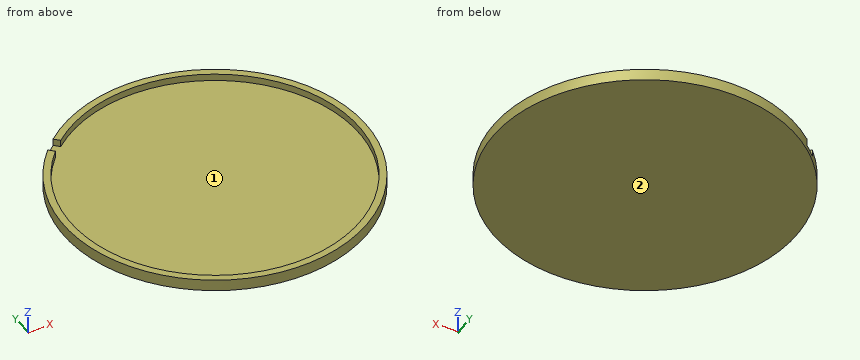
Autodesk Fusion 360 part; units mm, degrees
sketch "Sketch1" plane through (0, 0, 0) normal (0, 0, 1) x (1, 0, 0)
  circle A0 centre (0, 0) radius 65
  dimension "d1" = 130
extrude "Extrude1" add sketch "Sketch1" along normal blind 5
hole "Hole1" at (0, 0, 5) direction (0, 0, -1) diameter 124 depth 3 tip angle 180
sketch "Sketch2" plane through (0, 0, 5) normal (0, 0, 1) x (-1, 0, 0)
  circle A0 centre (0, 0) radius 62
  circle A1 centre (0, 0) radius 65
  line L0 (54.116, -50.8938) -> (49.1662, -55.8435)
  line L1 (49.1662, -55.8435) -> (34.7966, -41.4739)
  line L2 (34.7966, -41.4739) -> (39.7463, -36.5241)
  line L3 (39.7463, -36.5241) -> (54.116, -50.8938)
  dimension "d7" = 7
extrude "Extrude2" cut sketch "Sketch2" against normal blind 3 contours A0 A1 L1 L3 picked at (41.6647, -47.2432)
Can you work these out from the model? Positions are in its coordinate system, mm. Face numbers are marked on the shaded views. Round coordinates to 2 decimals unless told otherwise and drop trailing zeros. Write each loop counter-clockwise with the first axis right and the second up, starting at its lowest first coordinate (ties: lowest second). Pieces come first, ordered by that corner, then holes. Notation, with made-up numbers: M -35.5,15 L 2.5,15 A23 ccw 2.5,26 Z; hole C 36,-30.5 d2. An arc over 180 degrees is marked long. Use a Markdown table: item, result.
Item 1: We'd pull the mould along Y, two halves only. Please class the marked faces 1 and 2: released by +Y, released by -Y, zero draft, split by the parting line, or undercut.
Found:
| item | result |
|---|---|
| face 1 | undercut |
| face 2 | zero draft |
Item 2: I want a section at B-B (x = 35). List the corners of the cut face in (y, z) for me, and give its area (3 significant figures).
Found:
| item | result |
|---|---|
| outline | M -54.77,0 L 54.77,0 L 54.77,5 L 51.18,5 L 51.18,2 L -51.18,2 L -51.18,5 L -54.77,5 Z |
| area | 241 mm2 |
Item 3: For pin 1 Ø2 at (y, z) = (21, 3) entering from +X; pin 2 Ø1 at (x, y) = (28.5, -9) entering from +Z; pin 3 Ø3 at (x, z) = (-43, 1.5) entering from +Y, each with a flat end and sliding along its axis, tell me the tip position at first contact or that it passes through.
Found:
| item | result |
|---|---|
| pin 1 | stops at x = 61.85 |
| pin 2 | stops at z = 2 |
| pin 3 | stops at y = 50.03 |
Item 4: I want a section at A-A (y = 0). List the corners of the cut face in (x, z) for me, and give its area (3 significant figures).
Found:
| item | result |
|---|---|
| outline | M -65,0 L 65,0 L 65,5 L 62,5 L 62,2 L -62,2 L -62,5 L -65,5 Z |
| area | 278 mm2 |
Item 5: If I drill on line 1 along Y through (x, z) = (0.5, 3.95); line 2 along Z through (x, y) = (-29, 47.5), over which ranges is the centre line in solid material (lowest first)? Write a range as [from, to].
Found:
| item | result |
|---|---|
| line 1 | y = [-65, -62], [62, 65] |
| line 2 | z = [0, 2] |
Item 6: I want a section at C-C (z = 2.8). List the corners of the cut face in (x, y) for me.
Found:
| item | result |
|---|---|
| outline | M -47.54,44.32 A65 ccw long -42.5,49.18 L -40.37,47.05 A62 cw long -45.42,42.2 Z |
